from build123d import *

# Parameters (mm, degrees)
F1_DEPTH = 5
F2_DEPTH = 40
F3_SIZE  = 3
F5_DEPTH = 3
F6_SIZE  = 1


with BuildPart() as f1:
    # F0 (on Top) → F1 (new body)
    with BuildSketch(Plane.XY):
        with BuildLine():
            Line((55, 56.0835413635), (0, 56.0835413635))
            Line((0, 56.0835413635), (0, 46.0835413635))
            Line((0, 46.0835413635), (21.9390119762, 46.0835413635))
            ThreePointArc((21.9390119762, 46.0835413635), (27.5, 51.6445293873), (33.0609880238, 46.0835413635))
            Line((33.0609880238, 46.0835413635), (55, 46.0835413635))
            Line((55, 46.0835413635), (55, 56.0835413635))
        make_face()
        with BuildLine():
            Line((21.9390119762, 46.0835413635), (0, 46.0835413635))
            Line((0, 46.0835413635), (0, 0))
            Line((0, 0), (5, 0))
            ThreePointArc((5, 0), (27.5, 22.5), (50, 0))
            Line((50, 0), (55, 0))
            Line((55, 0), (55, 46.0835413635))
            Line((55, 46.0835413635), (33.0609880238, 46.0835413635))
            ThreePointArc((33.0609880238, 46.0835413635), (27.5, 40.5225533396), (21.9390119762, 46.0835413635))
        make_face()
    extrude(amount=F1_DEPTH)

    # F0 (on Top) → F2 (join)
    with BuildSketch(Plane.XY):
        with BuildLine():
            ThreePointArc((50, 0), (27.5, 22.5), (5, 0))
            Line((5, 0), (10, 0))
            ThreePointArc((10, 0), (27.5, 17.5), (45, 0))
            Line((45, 0), (50, 0))
        make_face()
    extrude(amount=F2_DEPTH)

    # F3
    f3_edges = [f1.edges().sort_by_distance(p)[0] for p in [
        (21.939012, 46.083541, 5),
    ]]
    chamfer(f3_edges, length=F3_SIZE)

    # F4 (on face) → F5 (join)
    with BuildSketch(Plane.XY.offset(40)):
        with BuildLine():
            Line((50, 0), (55, 0))
            ThreePointArc((55, 0), (27.5, 27.5), (0, 0))
            Line((0, 0), (5, 0))
            ThreePointArc((5, 0), (27.5, 22.5), (50, 0))
        make_face()
        with BuildLine():
            Line((45, 0), (50, 0))
            ThreePointArc((50, 0), (27.5, 22.5), (5, 0))
            Line((5, 0), (10, 0))
            ThreePointArc((10, 0), (27.5, 17.5), (45, 0))
        make_face()
        with BuildLine():
            Line((10, 0), (45, 0))
            ThreePointArc((45, 0), (27.5, 17.5), (10, 0))
        make_face()
    extrude(amount=F5_DEPTH)

    # F6
    f6_edges = [f1.edges().sort_by_distance(p)[0] for p in [
        (27.5, 27.5, 40),
    ]]
    chamfer(f6_edges, length=F6_SIZE)


solid = f1.part
Can you work these out from the model? Positions are in its coordinate system, mm. A direction names the side the tool comes from. Coordinates: 2 decimals unless noted, no trailing zeros. Order: outer loops, then holes, each group sorted by start corner. A loop starts at its lowest first (then second) coordinate and runs counter-clockwise, first axis right, second up. Notation, with made-up numbers: (19, -19.75) - (65, -19.75) arc R25 cw to (65, -2.75) - close; hole circle Ø6 at (33, -31.5). An arc over 180 degrees is marked (long way). Answer as a JSON object with one key per item and string values. Group by question number.
Q1. We'd pull the mould along X, two halves only. Please class faces 5 (the face through (55, 28, 2)), 6 (the face through (27, 35, 0)), 7 (the face through (27.995, 22.495, 22.255)), 8 (the face through (27, 7, 40)): +X half, -X half, draft (parallel to the pull), parting line (faces both ways), or undercut.
Q2. Imagine slicing it at A-A (x = 27.5). Please give me the cut outline in (y, z), and give its area (3 significant figures).
Q3. I need wall thicknesses on line 1 (Z direction, x = 51, y = 9.5); line 2 (Z direction, x = 38, y = 39); line 3 (Z direction, x = 42, y = 5.5). Which ranges of each line are inside material? Lowest first, please. Write a range as from..to.
Q4. On a 3-axis mill with a long thin cutter (end or side, diameter ignored), from which of +Z, -Z, +X, -X, +Y, -Y can I reach the whole of each face in a straight line? I mean faces 1 (the face through (27.115, 17.496, 19.72)), 2 (the face through (0, 28, 2)), 3 (the face through (28.105, 27.493, 41.986)), 4 (the face through (28.086, 26.653, 40.16)). Say none if no direction works.
Q5. Imagine slicing it at D-D (z = 17.5). Please give me the cut outline in (x, y).
Q6. Will these pins go through, and if not, where does the flat tip stop? P1, Ø6, axis at x = 24, z = 23, coming from the +Y side; P2, Ø3, axis at x = 43, y = 29, coming from the +Z side; P3, Ø3, axis at x = 43.5, z = 8, coming from the +Y side.
Q7. Imagine slicing it at C-C (y = 30.5). Please give me the cut outline in (x, z).
Q8. Imagine slicing it at B-B (z = 3). Please give me the cut outline in (x, y).
Determined:
{
 "1": {"face 5": "+X half", "face 6": "draft", "face 7": "parting line", "face 8": "undercut"},
 "2": {"outline": "(0, 40) - (17.5, 40) - (17.5, 0) - (40.52, 0) - (40.52, 2) - (37.52, 5) - (22.5, 5) - (22.5, 40) - (26.5, 40) - (27.5, 41) - (27.5, 43) - (0, 43) - close; (51.64, 0) - (56.08, 0) - (56.08, 5) - (54.64, 5) - (51.64, 2) - close", "area": "385 mm2"},
 "3": {"line 1": "z = 0..5, 40..43", "line 2": "z = 0..5", "line 3": "z = 40..43"},
 "4": {"face 1": "-Z, -Y", "face 2": "+Z, -Z, -X, +Y, -Y", "face 3": "+Z, +Y", "face 4": "+Y"},
 "5": {"outline": "(5, 0) - (10, 0) arc R17.5 cw to (45, 0) - (50, 0) arc R22.5 ccw to start"},
 "6": {"P1": "stops at y = 22.49", "P2": "stops at z = 5", "P3": "stops at y = 17.2"},
 "7": {"outline": "(0, 0) - (55, 0) - (55, 5) - (0, 5) - close"},
 "8": {"outline": "(0, 0) - (10, 0) arc R17.5 cw to (45, 0) - (55, 0) - (55, 56.08) - (0, 56.08) - close; hole circle Ø13.12 at (27.5, 46.08)"}
}
